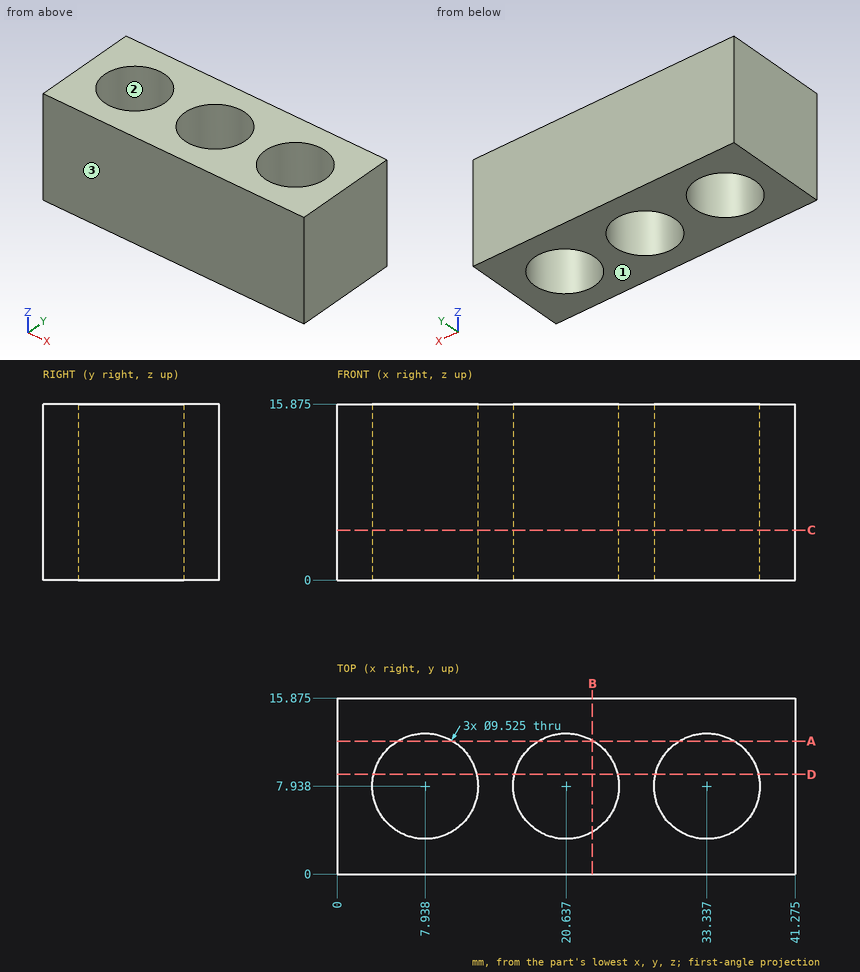
Check sheet for the drawn part. Datum: minimum x, y, z corner. Units: mm. Give positions to 0.01 mm unless a question says otherwise; leave off trailing zeros. Order: outer loops, then holes, each group sorted by start corner. A loop starts at its lowest first (then second) coordinate and runs counter-clockwise, first axis right, second up. Notation, with made-up numbers: (-32, 21.5) -> (-5, 21.5) arc R22 cw to (-5, 47.5) -> close; hole circle Ø6 at (37, 8). An arc over 180 degrees is marked (long way). Answer as CSV lines item,"result".
Q1. Sectioned sample at D-D on y = 9. Record the cut outline in (x, z) (1 decimal), plus the area to 3 significant figures.
Solutions:
outline,"(0, 0) -> (3.3, 0) -> (3.3, 15.9) -> (0, 15.9) -> close; (12.6, 0) -> (16, 0) -> (16, 15.9) -> (12.6, 15.9) -> close; (25.3, 0) -> (28.7, 0) -> (28.7, 15.9) -> (25.3, 15.9) -> close; (38, 0) -> (41.3, 0) -> (41.3, 15.9) -> (38, 15.9) -> close"
area,"213 mm²"
Q2. Sectioned sample at B-B on x = 23. Record the cut outline in (y, z) (1 decimal), plus the area to 3 significant figures.
Solutions:
outline,"(0, 0) -> (3.8, 0) -> (3.8, 15.9) -> (0, 15.9) -> close; (12.1, 0) -> (15.9, 0) -> (15.9, 15.9) -> (12.1, 15.9) -> close"
area,"121 mm²"
Q3. Sectioned sample at A-A on y = 12. Record the cut outline in (x, z) (1 decimal).
Solutions:
outline,"(0, 0) -> (5.5, 0) -> (5.5, 15.9) -> (0, 15.9) -> close; (10.4, 0) -> (18.2, 0) -> (18.2, 15.9) -> (10.4, 15.9) -> close; (23.1, 0) -> (30.9, 0) -> (30.9, 15.9) -> (23.1, 15.9) -> close; (35.8, 0) -> (41.3, 0) -> (41.3, 15.9) -> (35.8, 15.9) -> close"
Q4. Scan lines: probe 1 along Y at (x, z) = (33.5, 2.5) (1 decimal); probe 2 along X at (y, z) = (6, 10.5) (1 decimal); probe 3 along X at (y, z) = (5.5, 13.75) (1 decimal). Record each from-to range of solid material in increasing order.
Solutions:
probe 1,"y = 0 to 3.2, 12.7 to 15.9"
probe 2,"x = 0 to 3.6, 12.3 to 16.3, 25 to 29, 37.7 to 41.3"
probe 3,"x = 0 to 3.8, 12 to 16.5, 24.7 to 29.2, 37.4 to 41.3"
Q5. Release check for a two-part mould opening along Y. For the marked faces 1, 2 and 3 record: +Y half, -Y half, draft (parallel to the pull), parting line (faces both ways), or undercut.
Solutions:
face 1,"draft"
face 2,"undercut"
face 3,"-Y half"
Q6. Depth check by flat-ended pin: pin 1 (7.5 mm diameter, centred on x = 7.94, y = 7.94, fed in from +Z). Enter the tip coordinate at first touch or a pass-through.
Solutions:
pin 1,"passes through"
Q7. Sectioned sample at C-C on z = 4.5. Record the cut outline in (x, y) (1 decimal).
Solutions:
outline,"(0, 0) -> (41.3, 0) -> (41.3, 15.9) -> (0, 15.9) -> close; hole circle Ø9.5 at (7.9, 7.9); hole circle Ø9.5 at (20.6, 7.9); hole circle Ø9.5 at (33.3, 7.9)"
